Geometry check sheet. Reference: drawing and pictorial views, mm from the part's lowest x, y, z. A direction names the side the tool comes from. Coordinates: 2 decimals unless noted, no trailing zeros. Write each loop counter-clockwise with the first axis right and the second up, starting at its lowest first coordinate (ties: lowest second). Pieces come first, ordered by that corner, then holes. Notation, with made-up numbers: (5.25, 28.5) -> (22.25, 28.5) arc R16 ccw to (22.25, 39.5) -> close; hole circle Ø4 at (75, 29). An arc over 180 degrees is marked (long way). Put each result on its own line as item: value.
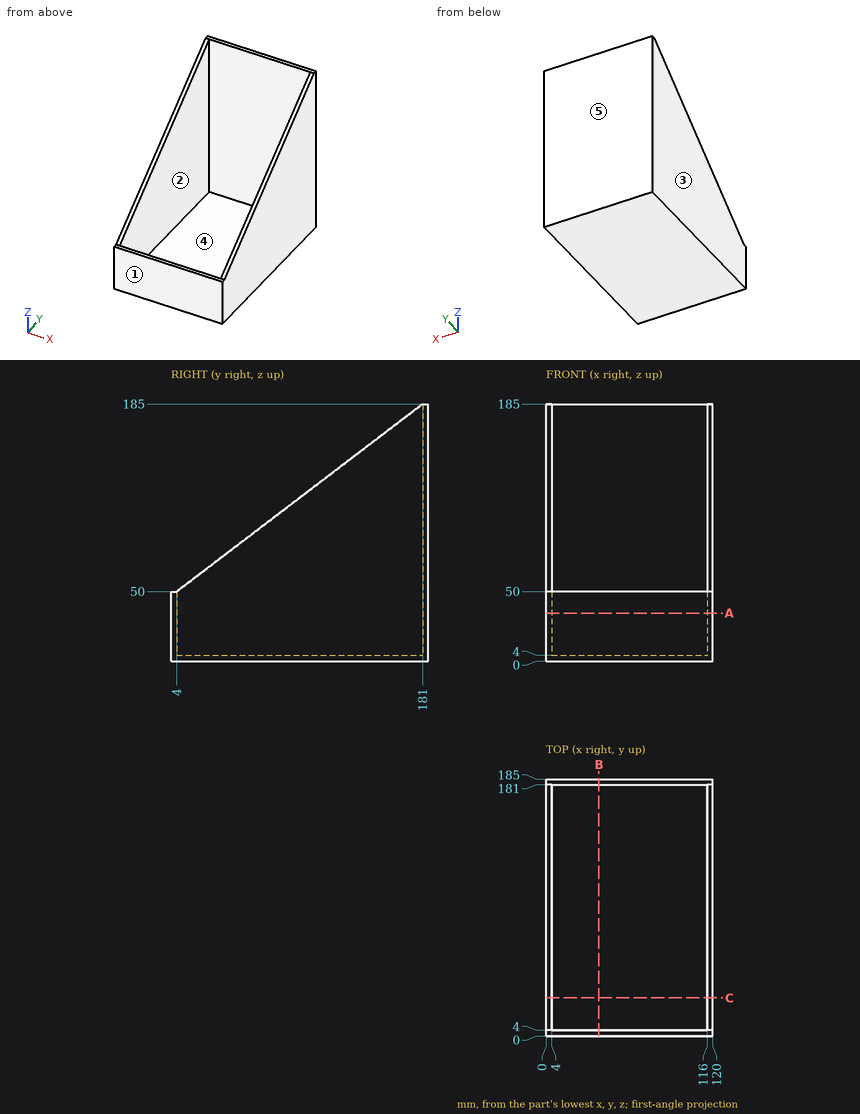
Q1. Material ranges on line 1 along Y through (x, z) = (22, 17); line 2 along X through (y, z) = (122, 49); line 3 along Z through (x, y) = (10, 33), recorded low to high.
Recorded:
line 1: y = 0 to 4, 181 to 185
line 2: x = 0 to 4, 116 to 120
line 3: z = 0 to 4
Q2. Cross-section at B-B (x = 38). Record the cut outline in (y, z).
Recorded:
outline: (0, 0) -> (185, 0) -> (185, 185) -> (181, 185) -> (181, 4) -> (4, 4) -> (4, 50) -> (0, 50) -> close
Q3. Mould release check, pull along X, two halves, no side actions. Record for the marked faces 3, 4 and 5: released by +X, released by -X, zero draft, split by the parting line, or undercut.
Recorded:
face 3: released by -X
face 4: undercut
face 5: zero draft
Q4. Tool access check on the marked faces 1 and 2. Record the directions out of +Z, -Z, +X, -X, +Y, -Y that give a thin tool (end or side, any length) a straight path to the whole face; none if there is none.
Recorded:
face 1: +Z, -Z, +X, -X, -Y
face 2: +Z
Q5. Cross-section at A-A (z = 34.5). Record the cut outline in (x, y), plus the area to 3 significant figures.
Recorded:
outline: (0, 0) -> (120, 0) -> (120, 185) -> (0, 185) -> close; hole (4, 4) -> (116, 4) -> (116, 181) -> (4, 181) -> close
area: 2,380 mm2
Q6. Cross-section at C-C (y = 27.5). Record the cut outline in (x, z).
Recorded:
outline: (0, 0) -> (120, 0) -> (120, 67.92) -> (116, 67.92) -> (116, 4) -> (4, 4) -> (4, 67.92) -> (0, 67.92) -> close
Q7. Depth check by flat-ended pin: P1, Ø4, axis at x = 68, y = 64.5, coming from the +Z side; P2, Ø1.2, axis at x = 62.5, y = 2, coming from the +Z side; P3, Ø4, axis at x = 98, z = 95, coming from the -Y side. Enter the tip coordinate at first touch or a pass-through.
Recorded:
P1: stops at z = 4
P2: stops at z = 50
P3: stops at y = 181
